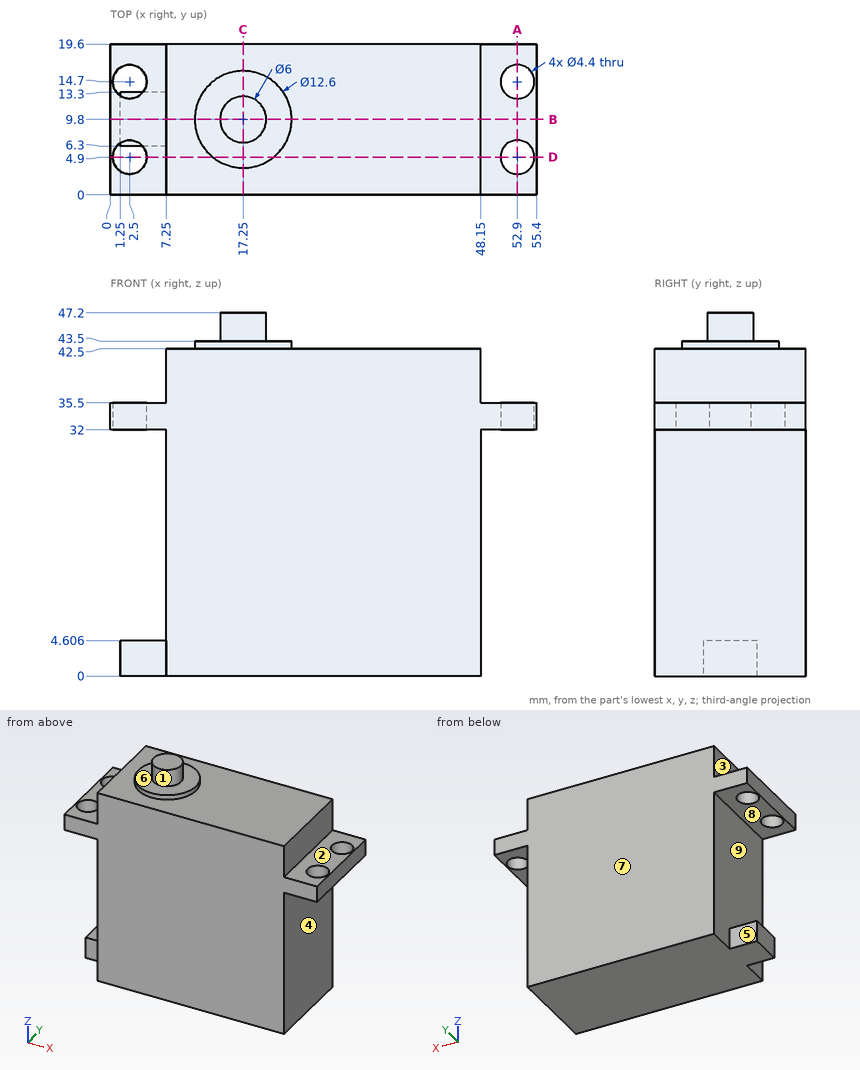
Geometry check sheet. Reference: drawing and pictorial views, mm from the part's lowest x, y, z. A direction names the side the tool comes from. Round coordinates to 2 decimals unless told otherwise and drop trailing zeros. Write each loop counter-clockwise with the first axis right and the second up, starting at its lowest first coordinate (ties: lowest second). Pieces come first, ordered by that corner, then holes. Notation, with made-up numbers: (32.25, 78) -> (41.25, 78) arc R22 cw to (41.25, 116) -> close; hole circle Ø5 at (53.25, 66). An arc over 180 degrees is marked (long way). Put each result on its own line as item: value.
1) Cross-section at A-A, the plane x = 52.9. Enter the section's corners in (y, z).
Recorded:
outline: (0, 32) -> (2.7, 32) -> (2.7, 35.5) -> (0, 35.5) -> close; (7.1, 32) -> (12.5, 32) -> (12.5, 35.5) -> (7.1, 35.5) -> close; (16.9, 32) -> (19.6, 32) -> (19.6, 35.5) -> (16.9, 35.5) -> close
2) Access from +Z, -Z, +X, -X, +Y, -Y to the whole of each face (thin tool, end or side, straight path). Record for the marked faces 1, 2, 3, 4 and 5.
Recorded:
face 1: +Z
face 2: +Z, +X, +Y, -Y
face 3: +Z, -X, +Y, -Y
face 4: -Z, +X, +Y, -Y
face 5: -Z, -X, +Y
3) Thickness scan on probe 1 along Y at (x, z) = (52.9, 34.1); probe 2 along Z at (x, y) = (23, 3); probe 3 along X at (y, z) = (15.5, 20). Record the ranges inside material, lowest first. Write a range as from..to.
Recorded:
probe 1: y = 0..2.7, 7.1..12.5, 16.9..19.6
probe 2: z = 0..42.5
probe 3: x = 7.25..48.15
4) Release check for a two-part mould opening along Z. For the marked faces 6, 7, 8 and 9 record: pulls with the +Z half, pulls with the -Z half, needs draft (parallel to the pull), parting line crosses it, or undercut.
Recorded:
face 6: pulls with the +Z half
face 7: needs draft
face 8: undercut
face 9: undercut
5) Cross-section at D-D, the plane y = 4.9. Enter the section's corners in (x, z), plus the area to 3 significant figures.
Recorded:
outline: (0, 32) -> (0.3, 32) -> (0.3, 35.5) -> (0, 35.5) -> close; (4.7, 32) -> (7.25, 32) -> (7.25, 0) -> (48.15, 0) -> (48.15, 32) -> (50.7, 32) -> (50.7, 35.5) -> (48.15, 35.5) -> (48.15, 42.5) -> (21.21, 42.5) -> (21.21, 43.5) -> (13.29, 43.5) -> (13.29, 42.5) -> (7.25, 42.5) -> (7.25, 35.5) -> (4.7, 35.5) -> close; (55.1, 32) -> (55.4, 32) -> (55.4, 35.5) -> (55.1, 35.5) -> close
area: 1,770 mm2
6) Cross-section at C-C, the plane x = 17.25. Enter the section's corners in (y, z), plus the area to 3 significant figures.
Recorded:
outline: (0, 0) -> (19.6, 0) -> (19.6, 42.5) -> (16.1, 42.5) -> (16.1, 43.5) -> (12.8, 43.5) -> (12.8, 47.2) -> (6.8, 47.2) -> (6.8, 43.5) -> (3.5, 43.5) -> (3.5, 42.5) -> (0, 42.5) -> close
area: 868 mm2
7) Cross-section at B-B, the plane y = 9.8. Enter the section's corners in (x, z), plus the area to 3 significant figures.
Recorded:
outline: (0, 32) -> (7.25, 32) -> (7.25, 4.61) -> (1.25, 4.61) -> (1.25, 0) -> (48.15, 0) -> (48.15, 32) -> (55.4, 32) -> (55.4, 35.5) -> (48.15, 35.5) -> (48.15, 42.5) -> (23.55, 42.5) -> (23.55, 43.5) -> (20.25, 43.5) -> (20.25, 47.2) -> (14.25, 47.2) -> (14.25, 43.5) -> (10.95, 43.5) -> (10.95, 42.5) -> (7.25, 42.5) -> (7.25, 35.5) -> (0, 35.5) -> close
area: 1,850 mm2
8) Depth check by flat-ended pin: P1, Ø2, axis at y = 8, z = 38.5, coming from the -X side; P2, Ø3.5, axis at x = 4, y = 6, coming from the +Z side; P3, Ø10, axis at x = 31, y = 14.5, coming from the +Z side. Enter the tip coordinate at first touch or a pass-through.
Recorded:
P1: stops at x = 7.25
P2: stops at z = 35.5
P3: stops at z = 42.5
